The model under review builds one solid part; all positions refer to its coordinate system, in mm. A direction names the side the tool comes from. Round coordinates to 2 decimals unless told otherwise and drop trailing zeros. Write each loop counter-clockwise with the first axis right and the second up, starting at its lowest first coordinate (ties: lowest second). Pieces come first, ordered by that corner, then holes.
Item 1: Draft analysis for pull direction Y (two halves, no side actions). For faces 1 (the face through (17, 50, 48)), 2 (the face through (75, 50, 1)), 3 (the face through (52.14, 72.27, -37.47)), state which applies: +Y half, -Y half, draft (parallel to the pull), parting line (faces both ways), or undercut.
Item 2: Machinability: for faces 4 (the face through (34.5, 50, 1)), 5 (the face through (-1, 50, 50)), which of the approach directions +Z, -Z, +X, -X, +Y, -Y give a long, thin tool a straight path to every point of the face, cutting with its end or side? Answer none if there is none.
Item 3: To check wall thickness, follow L1, parallel to Y at x = 17, z = 33.5; L2, parallel to Z at x = -50.5, y = 63; L3, parallel to Y at x = 17, z = -36.3. State the ranges of each line that lie inside material, in increasing order.
Item 4: Add section B-B (z = -33). State how many separate pieces and enclosed holes the cut face has, plus the area to 3 significant figures.
Item 5: Add section A-A (x = -41). Give the boundary of the cut face in (y, z), plus the area to 3 significant figures.
```python
from build123d import *

# Parameters (mm, degrees)
SKETCH1_W           = 150
SKETCH1_H           = 100
BOSS_EXTRUDE1_DEPTH = 100
SHELL1_T            = -2
SKETCH3_W           = 73
SKETCH3_H           = 2
SKETCH3_W_2         = 2
SKETCH3_H_2         = 96
EXTRUDE_THIN1_DEPTH = 98
SKETCH4_R           = 15
SKETCH4_R_2         = 13.5
BOSS_EXTRUDE2_DEPTH = 75
SKETCH6_R           = 6.25
SKETCH7_R           = 6.25
SKETCH11_R          = 6.25
SKETCH11_R_2        = 5
BOSS_EXTRUDE3_DEPTH = 5
SKETCH12_R          = 6.25
BOSS_EXTRUDE4_DEPTH = 5
SKETCH13_W          = 150
SKETCH13_H          = 100
BOSS_EXTRUDE5_DEPTH = 2


with BuildPart() as part:
    # Sketch1 → Boss-Extrude1 (new body)
    with BuildSketch(Plane(origin=(0, 0, 0), x_dir=(1, 0, 0), z_dir=(0, 1, 0))):
        Rectangle(SKETCH1_W, SKETCH1_H)
    extrude(amount=BOSS_EXTRUDE1_DEPTH)

    # Shell1
    shell1_openings = [part.faces().sort_by_distance(p)[0] for p in [
        (0, 100, 0),
    ]]
    offset(amount=SHELL1_T, openings=shell1_openings, kind=Kind.INTERSECTION)

    # Sketch3 → Extrude-Thin1 (add, through all)
    with BuildSketch(Plane(origin=(0, 2, 0), x_dir=(1, 0, 0), z_dir=(0, 1, 0))):
        with Locations((-36.5, -1)):
            Rectangle(SKETCH3_W, SKETCH3_H)
        with Locations((-55.75, 0)):
            Rectangle(SKETCH3_W_2, SKETCH3_H_2)
        with Locations((-37.5, 0)):
            Rectangle(SKETCH3_W_2, SKETCH3_H_2)
        with Locations((-1, 0)):
            Rectangle(SKETCH3_W_2, SKETCH3_H_2)
        with Locations((-19.25, 0)):
            Rectangle(SKETCH3_W_2, SKETCH3_H_2)
        with Locations((35.5, 0)):
            Rectangle(SKETCH3_W_2, SKETCH3_H_2)
    extrude(amount=EXTRUDE_THIN1_DEPTH)

    # Sketch4 → Boss-Extrude2 (add)
    # profile 1 of 4: a face of its own
    with BuildSketch(Plane(origin=(0, 0, 48), x_dir=(-1, 0, 0), z_dir=(0, 0, -1))):
        with Locations((-17, 67)):
            Circle(SKETCH4_R)
        with Locations((-17, 67)):
            Circle(SKETCH4_R_2, mode=Mode.SUBTRACT)
    # profile 2 of 4: a face of its own
    with BuildSketch(Plane(origin=(0, 0, 48), x_dir=(-1, 0, 0), z_dir=(0, 0, -1))):
        with Locations((-55.5, 67)):
            Circle(SKETCH4_R)
        with Locations((-55.5, 67)):
            Circle(SKETCH4_R_2, mode=Mode.SUBTRACT)
    # profile 3 of 4: a face of its own
    with BuildSketch(Plane(origin=(0, 0, 48), x_dir=(-1, 0, 0), z_dir=(0, 0, -1))):
        with Locations((-17, 22)):
            Circle(SKETCH4_R)
        with Locations((-17, 22)):
            Circle(SKETCH4_R_2, mode=Mode.SUBTRACT)
    # profile 4 of 4: a face of its own
    with BuildSketch(Plane(origin=(0, 0, 48), x_dir=(-1, 0, 0), z_dir=(0, 0, -1))):
        with Locations((-55.5, 22)):
            Circle(SKETCH4_R)
        with Locations((-55.5, 22)):
            Circle(SKETCH4_R_2, mode=Mode.SUBTRACT)
    extrude(amount=BOSS_EXTRUDE2_DEPTH)

    # Sketch6 → section 0 of loft2
    with BuildSketch(Plane.XY.offset(-35), mode=Mode.PRIVATE) as loft2_s0:
        with Locations((17, 67)):
            Circle(SKETCH6_R)
    # loft up to a face of the part (loft2)
    loft([loft2_s0.sketch, Face(Wire([part.edges().sort_by_distance((27.268206589, 77.934529411, -27))[0]]))])

    # Sketch7 → section 1 of loft3
    with BuildSketch(Plane.XY.offset(-35), mode=Mode.PRIVATE) as loft3_s1:
        with Locations((55.5, 67)):
            Circle(SKETCH7_R)
    # loft up to a face of the part (loft3)
    loft([Face(Wire([part.edges().sort_by_distance((65.768206589, 77.934529411, -27))[0]])), loft3_s1.sketch])

    # Sketch11 → Boss-Extrude3 (add)
    with BuildSketch(Plane(origin=(0, 0, -35), x_dir=(-1, 0, 0), z_dir=(0, 0, -1))):
        with Locations((-17, 67)):
            Circle(SKETCH11_R)
        with Locations((-17, 67)):
            Circle(SKETCH11_R_2, mode=Mode.SUBTRACT)
    extrude(amount=BOSS_EXTRUDE3_DEPTH)

    # Sketch12 → Boss-Extrude4 (add)
    with BuildSketch(Plane(origin=(0, 0, -35), x_dir=(-1, 0, 0), z_dir=(0, 0, -1))):
        with Locations((-55.5, 67)):
            Circle(SKETCH12_R)
    extrude(amount=BOSS_EXTRUDE4_DEPTH)

    # Sketch13 → Boss-Extrude5 (add)
    with BuildSketch(Plane(origin=(0, 100, 0), x_dir=(1, 0, 0), z_dir=(0, 1, 0))):
        Rectangle(SKETCH13_W, SKETCH13_H)
    extrude(amount=BOSS_EXTRUDE5_DEPTH)


solid = part.part
```
Numbers:
1. face 1: undercut
1. face 2: draft
1. face 3: undercut
2. face 4: none
2. face 5: +Z, +X, -X, +Y, -Y
3. L1: y = 0 to 2, 7 to 8.5, 35.5 to 37, 52 to 53.5, 80.5 to 82, 100 to 102
3. L2: z = -50 to -48, 0 to 2, 48 to 50
3. L3: y = 0 to 2, 60.75 to 62, 72 to 73.25, 100 to 102
4. separate pieces: 3
4. enclosed holes: 6
4. area: 2,420 mm2
5. outline: (0, -50) - (102, -50) - (102, 50) - (0, 50) - close; hole (2, -48) - (100, -48) - (100, 0) - (2, 0) - close; hole (2, 2) - (100, 2) - (100, 48) - (2, 48) - close
5. area: 988 mm2
